Autodesk Fusion 360 part; units mm, degrees
sketch "Sketch1" plane through (0, 0, 0) normal (0, 0, 1) x (1, 0, 0)
  circle A0 centre (0, 0) radius 15.65
  circle A1 centre (0, 0) radius 18.9
  dimension "d3" = 31.3
  dimension "d11" = 37.8
extrude "Extrude1" add sketch "Sketch1" along normal blind 3 contours A0
sketch "Sketch2" plane through (0, 0, 3) normal (0, 0, 1) x (-1, 0, 0)
  circle A0 centre (0, 0) radius 15.65
  line L0 (-5, -18) -> (5, -18)
  line L1 (5, -18) -> (5, 18)
  line L2 (5, 18) -> (-5, 18)
  line L3 (-5, 18) -> (-5, -18)
  line L4 (-5, -18) -> (5, 18) construction
  line L5 (5, -18) -> (-5, 18) construction
  dimension "d7" = 10
  dimension "d8" = 36
extrude "Extrude2" add sketch "Sketch2" along normal blind 1.5 contours A0 L1 L3 | A0 L1 L2 L3 | A0 L0 L1 L3
extrude "Extrude3" add sketch "Sketch1" against normal blind 2 contours A0 | A1
equation "bigID = 31.3 mm"
equation "bigtab = 36 mm"
equation "d3 = bigID"
equation "bigtabwidth = 10 mm"
equation "d7 = bigtabwidth"
equation "d8 = bigtab"
equation "d11 = bigID + 6.5 mm"
Verification items for the finished model (mm, model axes). A direction names the side the tool comes from. Give positions to 0.01 mm unless a question says otherwise; leave off trailing zeros. Order: outer loops, then holes, each group sorted by start corner. A loop starts at its lowest first (then second) coordinate and runs counter-clockwise, first axis right, second up. Notation, with made-up numbers: M 36,42.5 L 59,42.5 A22 ccw 59,67.5 Z; hole C 81.25,-22.75 d5. An arc over 180 degrees is marked long. Answer as a JSON object with one key per item and string values. Group by question number.
1) Cross-section at A-A (x = 0). Enter the section's corners in (y, z).
2) Depth check by flat-ended pin: pin 1 Ø1.2 at (x, z) = (-0.5, 3.5) entering from +Y; pin 2 Ø0.8 at (y, z) = (1.5, 4) entering from -X; pin 3 Ø3 at (x, y) = (14, -0.5) entering from +Z. Enter the tip coordinate at first touch or a pass-through.
3) Cross-section at D-D (x = -7). Enter the section's corners in (y, z), then the cut area to 3 significant figures.
4) Cross-section at B-B (y = 0). Enter the section's corners in (x, z).
5) Scan lines: line 1 along Z through (x, y) = (12.5, -7); line 2 along Z through (x, y) = (-10, 12.5); line 3 along X through (y, z) = (-9, 3.5). Record each from-to range of solid material in increasing order. Write a range as [from, to].
6) Access from +Z, -Z, +X, -X, +Y, -Y to the whole of each face (thin tool, end or side, straight path). Record for faces 4 (the face through (-9, 0, 3)), 5 (the face through (5, 0, 4)), 6 (the face through (0, -18, 4)).
7) Cross-section at C-C (z = 3.5). Enter the section's corners in (x, y).
8) Mould release check, pull along Z, two halves, no side actions. Record for faces 1 (the face through (-2.037, -15.517, 1.479)), 2 (the face through (-5, 0, 4)), 3 (the face through (9, 0, 3)): released by +Z, released by -Z, zero draft, split by the parting line, or undercut.
Result sheet:
{
 "1": {"outline": "M -18.9,-2 L 18.9,-2 L 18.9,0 L 15.65,0 L 15.65,3 L 18,3 L 18,4.5 L -18,4.5 L -18,3 L -15.65,3 L -15.65,0 L -18.9,0 Z"},
 "2": {"pin 1": "stops at y = 18", "pin 2": "stops at x = -5", "pin 3": "stops at z = 3"},
 "3": {"outline": "M -17.56,-2 L 17.56,-2 L 17.56,0 L 14,0 L 14,3 L -14,3 L -14,0 L -17.56,0 Z", "area": "154 mm2"},
 "4": {"outline": "M -18.9,-2 L 18.9,-2 L 18.9,0 L 15.65,0 L 15.65,3 L 5,3 L 5,4.5 L -5,4.5 L -5,3 L -15.65,3 L -15.65,0 L -18.9,0 Z"},
 "5": {"line 1": "z = [-2, 3]", "line 2": "z = [-2, 0]", "line 3": "x = [-5, 5]"},
 "6": {"face 4": "+Z, -X, +Y, -Y", "face 5": "+Z, +X, +Y, -Y", "face 6": "+Z, +X, -X, -Y"},
 "7": {"outline": "M -5,-18 L 5,-18 L 5,18 L -5,18 Z"},
 "8": {"face 1": "undercut", "face 2": "zero draft", "face 3": "released by +Z"}
}
